Geometry check sheet. Reference: drawing and pictorial views, mm from the part's lowest x, y, z. A direction names the side the tool comes from. Give positions to 0.01 mm unless a question says otherwise; leave off trailing zeros. Write each loop counter-clockwise with the first axis right and the second up, starting at its lowest first coordinate (ties: lowest second). Pieces come first, ordered by that corner, then holes. Notation, with made-up numbers: (-22, 72) - (7, 72) arc R6 ccw to (7, 81) - close; hole circle Ø9 at (5.25, 79.5). An arc over 180 degrees is marked (long way). Put each result on its own line as item: value.
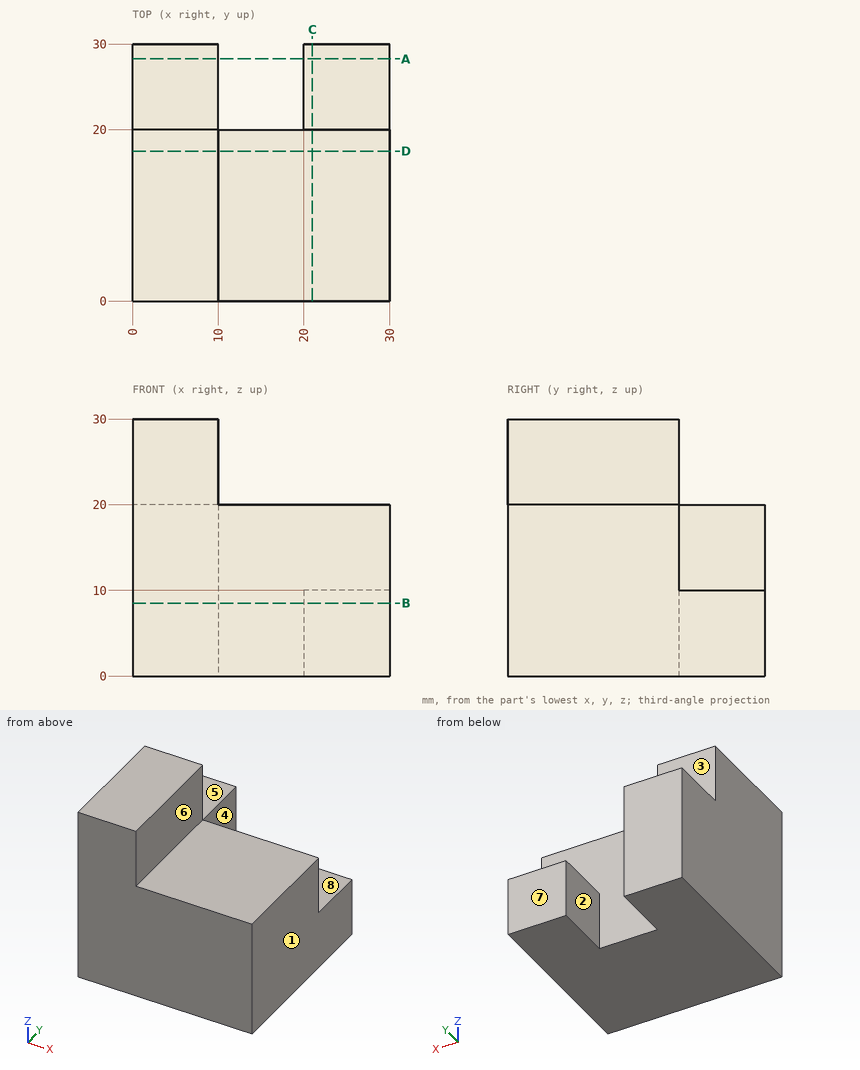
Q1. Set-up check for the marked faces 5, 6, 7 and 8: record each of +Z, -Z, +X, -X, +Y, -Y from which the full face is reachable in a straight line by a thin tool's end or side.
Answers follow:
face 5: +Z, +X, -X, +Y
face 6: +Z, +X, +Y, -Y
face 7: +Z, -Z, +X, -X, +Y
face 8: +Z, +X, +Y
Q2. Section check A-A, the plane y = 28.25. Record the cut outline in (x, z).
Answers follow:
outline: (0, 0) - (10, 0) - (10, 20) - (0, 20) - close; (20, 0) - (30, 0) - (30, 10) - (20, 10) - close
Q3. Section check D-D, the plane y = 17.5. Record the cut outline in (x, z).
Answers follow:
outline: (0, 0) - (30, 0) - (30, 20) - (10, 20) - (10, 30) - (0, 30) - close
Q4. Section check B-B, the plane z = 8.5. Record the cut outline in (x, y).
Answers follow:
outline: (0, 0) - (30, 0) - (30, 30) - (20, 30) - (20, 20) - (10, 20) - (10, 30) - (0, 30) - close
Q5. Go/stop test with flat-tipped pins: pin 1 Ø6 at (x, y) = (16.5, 12.5) entering from +Z; pin 2 Ø8 at (x, y) = (23.5, 27.5) entering from +Z; pin 3 Ø8 at (x, z) = (26.5, 15.5) entering from +Y. Record where each tip stops, or that it passes through.
Answers follow:
pin 1: stops at z = 20
pin 2: stops at z = 10
pin 3: stops at y = 20
Q6. Release check for a two-part mould opening along X. For the marked faces 1, 2, 3 and 4 record: released by +X, released by -X, zero draft, split by the parting line, or undercut.
Answers follow:
face 1: released by +X
face 2: undercut
face 3: zero draft
face 4: undercut
Q7. Scan lines: line 1 along Z through (x, y) = (14.25, 13.75); line 2 along X through (y, z) = (28.75, 16). Record each from-to range of solid material in increasing order.
Answers follow:
line 1: z = 0 to 20
line 2: x = 0 to 10
Q8. Section check C-C, the plane x = 21. Record the cut outline in (y, z), plus the area to 3 significant figures.
Answers follow:
outline: (0, 0) - (30, 0) - (30, 10) - (20, 10) - (20, 20) - (0, 20) - close
area: 500 mm2
